Input: dimensioned drawing with shaded views. Units: mm. Origin: part minimum x, y, z. A direction names the side the tool comes from. Round coordinates to 2 decimals unless told otherwise and drop trailing zeros. Order: outer loops, then holes, each group sorted by start corner. A loop starts at its lowest first (then second) coordinate and runs counter-clockwise, first axis right, second up. Notation, with made-up numbers: (67, 56) - (112, 56) arc R29 ccw to (112, 81) - close; hole circle Ø2 at (26, 41.25). An arc over 180 degrees is marked (long way). Return JSON: item names as keys, results as strings. Group by question number.
1) Section A-A, the plane y = 14.5. Return loops of the section in (x, z).
2) Section D-D, the plane y = 7.25. Return loops of the section in (x, z).
3) Contact query for flat-ended pins moving along their axis: P1, Ø1.5, axis at y = 25.5, z = 2.5, coming from the +X side (1 decimal); P2, Ø4, axis at x = 23, z = 1, coming from the +Y side; P3, Ø3, axis at x = 14.5, y = 15, coming from the -Z side; P4, Ø2.5, axis at x = 14.5, y = 14.5, coming from the +Z side. Output: stop coordinate, or through.
4) Section B-B, the plane z = 4.25. Return loops of the section in (x, y).
5) Ray query, line 1 (Y direction, x = 14.5, z = 5.75); line 2 (Z direction, x = 19.25, y = 22); line 3 (X direction, y = 14, z = 7.5) (1 decimal). Return the intervals inside material, ascending. Write a range as from..to.
6) Access query for the marked faces 1, 2 and 3. Directions: +Z, -Z, +X, -X, +Y, -Y. A direction counts if a zero-diameter tool reaches every point of the face in a straight line with its end or side. Return the directions, or none.
7) Mould query, pull axis X, two halves, no side actions, for the marked faces 4, 5 and 6. Classes: pulls with the +X half, pulls with the -X half, needs draft (parallel to the pull), parting line crosses it, or undercut.
8) Section C-C, the plane x = 12.5. Return loops of the section in (y, z).
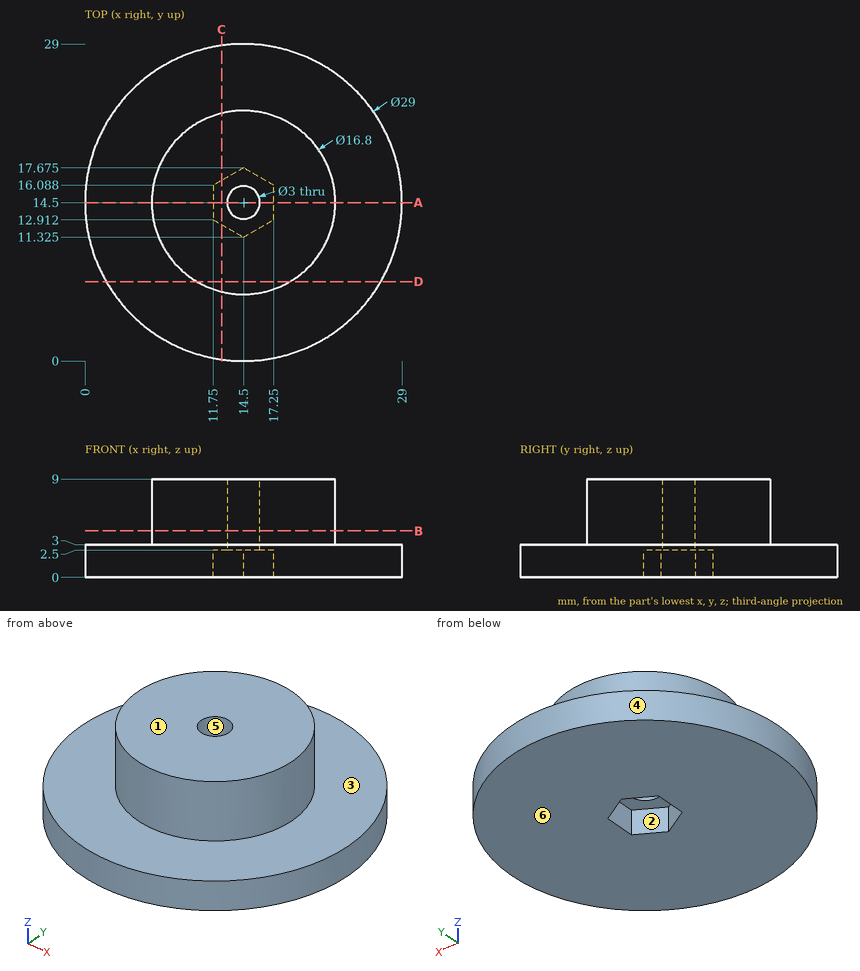
Geometry check:
{
 "1": {"outline": "(0, 0) - (11.75, 0) - (11.75, 2.5) - (13, 2.5) - (13, 9) - (6.1, 9) - (6.1, 3) - (0, 3) - close; (16, 2.5) - (17.25, 2.5) - (17.25, 0) - (29, 0) - (29, 3) - (22.9, 3) - (22.9, 9) - (16, 9) - close"},
 "2": {"outline": "(1.94, 0) - (27.06, 0) - (27.06, 3) - (18.74, 3) - (18.74, 9) - (10.26, 9) - (10.26, 3) - (1.94, 3) - close"},
 "3": {"P1": "x = 24.8", "P2": "y = 27.46", "P3": "z = 2.5", "P4": "through"},
 "4": {"outline": "circle Ø16.8 at (14.5, 14.5); hole circle Ø3 at (14.5, 14.5)"},
 "5": {"line 1": "6.1..13, 16..22.9", "line 2": "0..3", "line 3": "6.1..13.1, 15.9..22.9"},
 "6": {"face 1": "+Z, +X, -X, +Y, -Y", "face 2": "-Z", "face 3": "+Z"},
 "7": {"face 4": "parting line crosses it", "face 5": "undercut", "face 6": "needs draft"},
 "8": {"outline": "(0.14, 0) - (12.48, 0) - (12.48, 2.5) - (16.52, 2.5) - (16.52, 0) - (28.86, 0) - (28.86, 3) - (22.66, 3) - (22.66, 9) - (6.34, 9) - (6.34, 3) - (0.14, 3) - close"}
}
